from build123d import *

# Parameters (mm, degrees)
CHAMFER1_SIZE                   = 0.5
TAP_DRILL_FOR_M3X0_5_TAP1_D     = 2.5
TAP_DRILL_FOR_M3X0_5_TAP1_DEPTH = 6
TAP_DRILL_FOR_M3X0_5_TAP1_TIP   = 0.751075774


with BuildPart() as part:
    # Sketch1 → Revolve1 (revolve)
    with BuildSketch(Plane.XY):
        Polygon((0, 0), (23, 0), (23, 3), (15, 3), (15, 4), (9.8, 4), (9.8, 2.99), (0, 2.99), align=None)
    revolve(axis=Axis((0, 0, 0), (1, 0, 0)))

    # Chamfer1
    chamfer1_edges = [part.edges().sort_by_distance(p)[0] for p in [
        (23, -3, 0),
    ]]
    chamfer(chamfer1_edges, length=CHAMFER1_SIZE)

    # Tap Drill for M3x0.5 Tap1
    with Locations(Plane.ZY):
        with Locations((0, 0)):
            Hole(TAP_DRILL_FOR_M3X0_5_TAP1_D / 2, depth=TAP_DRILL_FOR_M3X0_5_TAP1_DEPTH)
            with Locations((0, 0, -(TAP_DRILL_FOR_M3X0_5_TAP1_DEPTH + TAP_DRILL_FOR_M3X0_5_TAP1_TIP / 2))):  # 118° drill point
                Cone(0, TAP_DRILL_FOR_M3X0_5_TAP1_D / 2, TAP_DRILL_FOR_M3X0_5_TAP1_TIP, mode=Mode.SUBTRACT)


solid = part.part
Model file for the job. Use its own axes, mm. A direction names the side the tool comes from. Coordinates: 2 decimals unless noted, no trailing zeros. Order: outer loops, then holes, each group sorted by start corner. A loop starts at its lowest first (then second) coordinate and runs counter-clockwise, first axis right, second up. Notation, with made-up numbers: M 78,-23 L 87,-23 A18 ccw 87,-19 Z; hole C 50,69.25 d11. An arc over 180 degrees is marked long. Return JSON: item names as keys, results as strings.
1. Flat gauge pins, fed straight in: pin 1 (2 mm diameter, centred on y = -2.5, z = 2.5, fed in from +X); pin 2 (1 mm diameter, centred on x = 5.5, z = -1, fed in from -Y); pin 3 (2 mm diameter, centred on y = 0, z = 0, fed in from -X). Where does each tip first touch, or does it go through?
Ans:
{"pin 1": "x = 22.96", "pin 2": "y = -2.95", "pin 3": "x = 6.15"}
2. Drill centre lines: probe 1 along Z at (x, y) = (2.45, 0); probe 2 along Z at (x, y) = (4.5, 0.75); probe 3 along X at (y, z) = (-1.75, -3.5). Where is each one in solid material? Low to high.
Ans:
{"probe 1": "-2.99 to -1.25, 1.25 to 2.99", "probe 2": "-2.89 to -1, 1 to 2.89", "probe 3": "9.8 to 15"}
3. Saw through at A-A (x = 1.5). Give the cut face in (y, z).
Ans:
{"outline": "C 0,0 d5.98; hole C 0,0 d2.5"}
4. Pull direction Z, two halves, no side cores. Call faces 1 (the face through (19, -3, 0)), 2 (the face through (0, 1, -1)), 3 (the face through (3.04, -1.22, 0.27)): +Z half, -Z half, draft (parallel to the pull), parting line (faces both ways), or undercut.
Ans:
{"face 1": "parting line", "face 2": "draft", "face 3": "undercut"}
5. Saw through at B-B (x = 9). Give the cut face in (y, z).
Ans:
{"outline": "C 0,0 d5.98"}
6. Saw through at D-D (x = 15.75). Give the cut face in (y, z), and give its area (3 significant figures).
Ans:
{"outline": "C 0,0 d6", "area": "28.3 mm^2"}
7. Saw through at C-C (z = -3.25). Give the cut face in (x, y), and give its area (3 significant figures).
Ans:
{"outline": "M 9.8,-2.33 L 15,-2.33 L 15,2.33 L 9.8,2.33 Z", "area": "24.3 mm^2"}
8. Tool access for faces 4 (the face through (12.364, -0.867, -3.905)), 5 (the face through (15, -1, 3)), 6 (the face through (9.8, 1, -3)): list every direction of +Z, -Z, +X, -X, +Y, -Y with a clear straight run to the whole face (end or side of a thin tool).
Ans:
{"face 4": "+X, -X", "face 5": "+X", "face 6": "-X"}
